Check sheet for the drawn part. Datum: minimum x, y, z corner. Units: mm. Give positions to 0.01 mm unless a question says otherwise; leave off trailing zeros. Loops run counter-clockwise (first coordinate to the right, second up) from the corner with the lowest first, then second, coordinate; pieces in that order, holes last.
1. Cross-section at B-B, the plane z = 14.5. Record the cut outline in (x, y).
2. Cross-section at A-A, the plane z = 8. Record the cut outline in (x, y) (3 decimals), plus the area to 3 significant figures.
3. Material ranges on L1, parallel to Y at x = 6.5, z = 12.5; L2, parallel to X at y = 1, z = 8 (3 decimals), recorded low to high.
4. Go/stop test with a flat-tipped pin: pin 1 Ø1.5 at (x, z) = (4.5, 10) entering from -Y. Record where the tip stops, or that it passes through.
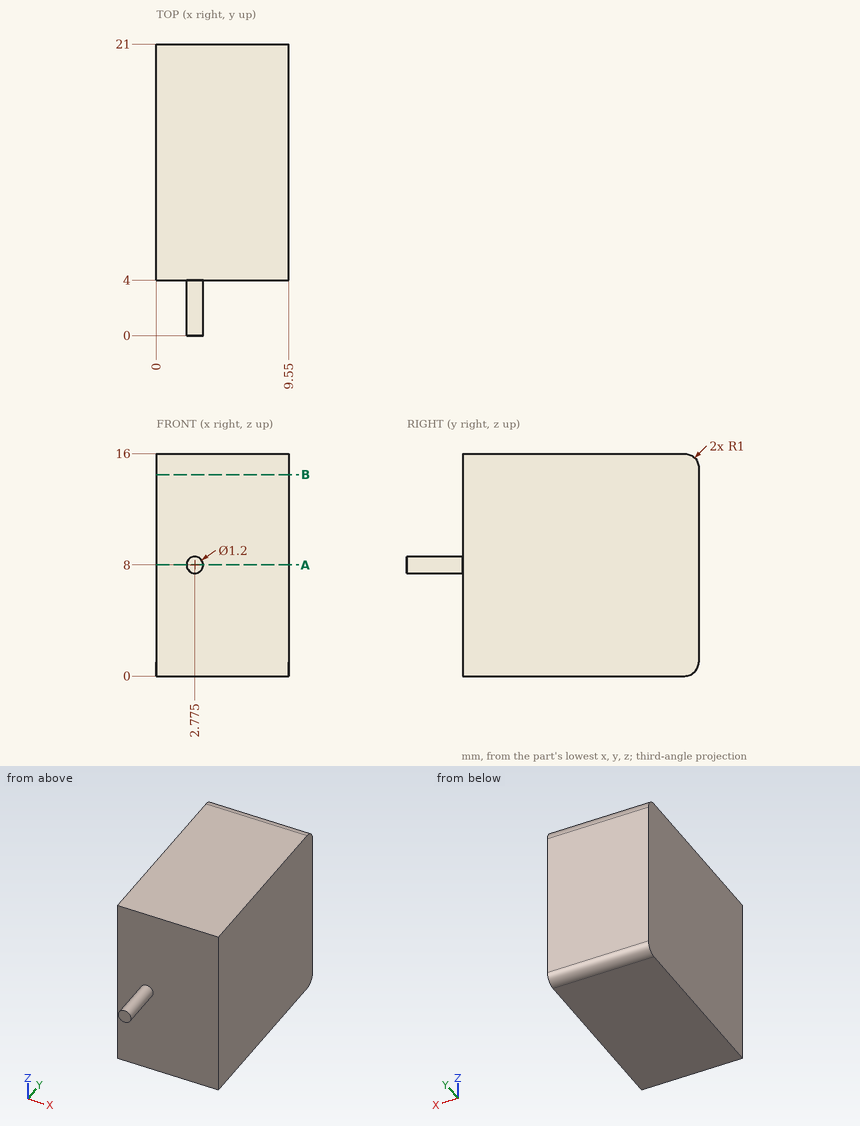
Result:
1. outline: (0, 4) - (9.55, 4) - (9.55, 21) - (0, 21) - close
2. outline: (0, 4) - (2.175, 4) - (2.175, 0) - (3.375, 0) - (3.375, 4) - (9.55, 4) - (9.55, 21) - (0, 21) - close
2. area: 167 mm2
3. L1: y = 4 to 21
3. L2: x = 2.175 to 3.375
4. pin 1: stops at y = 4
